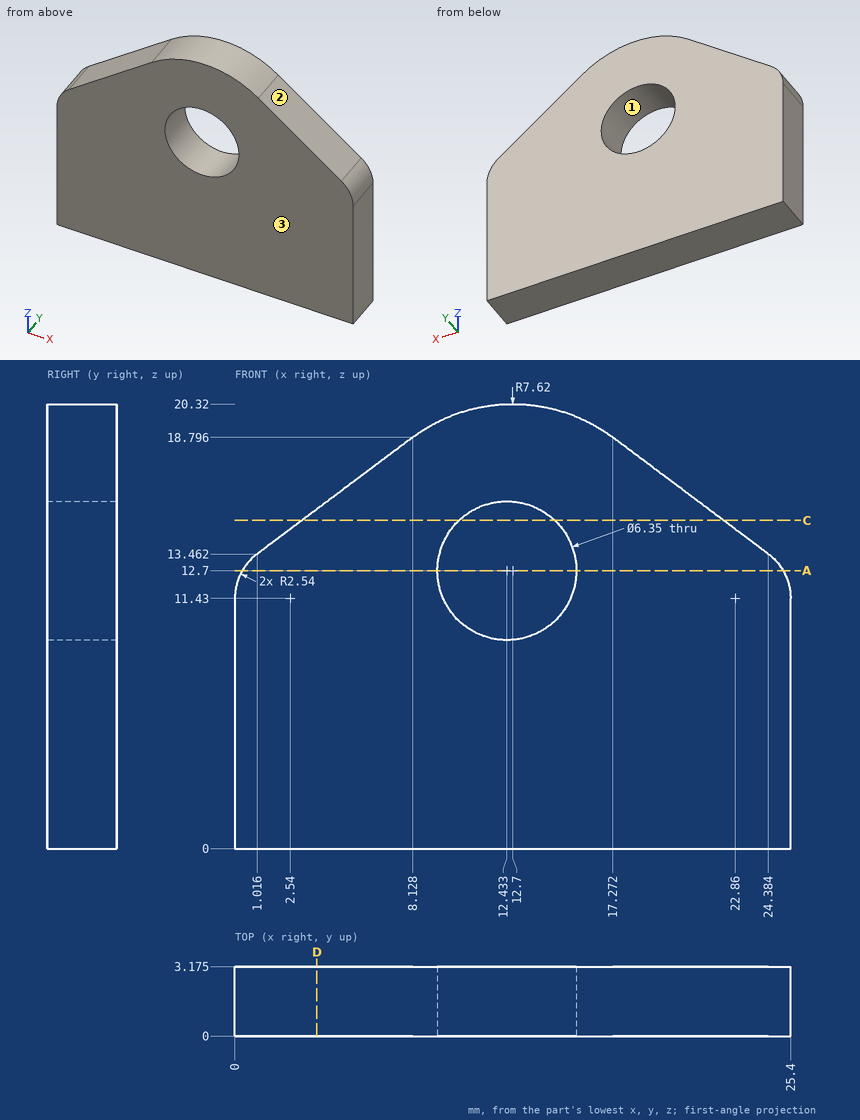
Can you work these out from the drawing? Everything is in mm from the part's minimum corner. Round coordinates to 2 decimals unless told otherwise and drop trailing zeros. Loops run counter-clockwise (first coordinate to the right, second up) from the corner with the lowest first, then second, coordinate; pieces in that order, holes last. Notation, with made-up numbers: M 14.5,30.5 L 26.5,30.5 A6 ccw 26.5,38.5 Z; hole C 56,89.5 d9. An arc over 180 degrees is marked long. Write item = value, one per line.
1. I want a section at D-D, the plane x = 3.75. Write out the boundary of the cut face in (y, z) (1 decimal).
Results below:
outline = M 0,0 L 3.2,0 L 3.2,15.5 L 0,15.5 Z
2. I want a section at C-C, the plane z = 15. Write out the boundary of the cut face in (x, y) (1 decimal).
Results below:
outline = M 3.1,0 L 10.2,0 L 10.2,3.2 L 3.1,3.2 Z; M 14.6,0 L 22.3,0 L 22.3,3.2 L 14.6,3.2 Z
3. I want a section at A-A, the plane z = 12.7. Write out the boundary of the cut face in (x, y) (1 decimal), and give its area (3 significant figures).
Results below:
outline = M 0.3,0 L 9.3,0 L 9.3,3.2 L 0.3,3.2 Z; M 15.6,0 L 25.1,0 L 25.1,3.2 L 15.6,3.2 Z
area = 58.3 mm²
4. I need wall thicknesses on probe 1 along X at (y, z) = (2.3, 12.7); probe 2 along X at (y, z) = (3.05, 14.75) (1 decimal); probe 3 along Z at (x, y) = (16.5, 2.95) (1 decimal). Which ranges of each line are inside material? Lowest first, please.
Results below:
probe_1 = 0.34 to 9.26, 15.61 to 25.06
probe_2 = 2.7 to 10, 14.9 to 22.7
probe_3 = 0 to 19.3
5. Thinking about a two-plate mould opening in X: for the marked faces 1, 2 and 3, which applies, +X half, -X half, draft (parallel to the pull), parting line (faces both ways), or undercut?
Results below:
face_1 = undercut
face_2 = +X half
face_3 = draft
